Autodesk Inventor part; units mm, degrees
ref_plane "YZ Plane" through (0, 0, 0) normal (1, 0, 0) x (0, 1, 0)
ref_plane "XZ Plane" through (0, 0, 0) normal (0, 1, 0) x (-1, 0, 0)
ref_plane "XY Plane" through (0, 0, 0) normal (0, 0, 1) x (1, 0, 0)
sketch "Sketch1" plane through (0, 0, 0) normal (0, 0, 1) x (1, 0, 0)
  circle A0 centre (0, 0) radius 4.725
  circle A1 centre (0, 0) radius 3
  circle A2 centre (0, 0) radius 4
  dimension "d0" = 9.45
  dimension "d1" = 6
  dimension "d4" = 8
extrude "Extrusion1" add sketch "Sketch1" along normal blind 1.55 contours A0 | A2
extrude "Extrusion2" add sketch "Sketch1" against normal blind 11.17 contours A2
chamfer "Chamfer1" distance 0.25 angle 45 1 edges at (-4.725, 0, 1.55)
properties part number "Tetrix Bronze Bushing (modified to fit vex couplers)" material "Bronze, Soft Tin"
Verification items for the finished model (mm, model axes). A direction names the side the tool comes from. Round coordinates to 2 decimals unless told otherwise and drop trailing zeros. Loops run counter-clockwise (first coordinate to the right, second up) from the corner with the lowest first, then second, coordinate; pieces in that order, holes last. Notation, with made-up numbers: (-19, 53.5) - (35, 53.5) arc R17 ccw to (35, 72.5) - close; hole circle Ø5 at (-34.5, 33.25). An arc over 180 degrees is marked (long way). Use a Markdown table: item, result. Add a question column.
1. Release check for a two-part mould opening along X. For faces 1 (the face through (-0.867, -3.905, -5.507)), 2 (the face through (-3, 0, -5)), 3 (the face through (1, 3, -11.17)) record: released by +X, released by -X, zero draft, split by the parting line, or undercut.
2. Access from +Z, -Z, +X, -X, +Y, -Y to the whole of each face (thin tool, end or side, straight path). Record for faces 4 (the face through (1, -3, 1.55)), 5 (the face through (-4, 2, 0)).
3. Thickness scan on probe 1 along Y at (x, z) = (0, -3); probe 2 along Z at (x, y) = (-1.25, 4); probe 3 along Y at (x, z) = (2.5, -2.75). Record the ranges inside material, lowest first. Write a range as [from, to].
4. Gauge pin test, flat ends, axial feed: pin 1 (3 mm diameter, centred on y = -0.5, z = -8, fed in from +X); pin 2 (1 mm diameter, centred on x = -3.5, z = -6.5, fed in from -Y); pin 3 (1.5 mm diameter, centred on y = 2, z = -3, fed in from +X). Record the tip position at first contact, or that the pin passes through.
5. Section check A-A, the plane x = 0. Record the boundary of the cut face in (y, z) (3 decimals).
6. Section check C-C, the plane z = -9.5. Record the boundary of the cut face in (x, y), plus the area to 3 significant figures.
Checks:
| question | item | result |
|---|---|---|
| 1 | face 1 | split by the parting line |
| 1 | face 2 | undercut |
| 1 | face 3 | zero draft |
| 2 | face 4 | +Z, +X, -X, +Y, -Y |
| 2 | face 5 | -Z |
| 3 | probe 1 | y = [-4, -3], [3, 4] |
| 3 | probe 2 | z = [0, 1.55] |
| 3 | probe 3 | y = [-3.12, -1.66], [1.66, 3.12] |
| 4 | pin 1 | stops at x = 4 |
| 4 | pin 2 | stops at y = -2.65 |
| 4 | pin 3 | stops at x = 3.8 |
| 5 | outline | (-4.725, 0) - (-4, 0) - (-4, -11.17) - (-3, -11.17) - (-3, 1.55) - (-4.475, 1.55) - (-4.725, 1.3) - close; (3, -11.17) - (4, -11.17) - (4, 0) - (4.725, 0) - (4.725, 1.3) - (4.475, 1.55) - (3, 1.55) - close |
| 6 | outline | circle Ø8 at (0, 0); hole circle Ø6 at (0, 0) |
| 6 | area | 22.0 mm^2 |
